```python
from build123d import *

# Parameters (mm, degrees)
BOSS_EXTRUDE1_DEPTH = 1
SKETCH2_W           = 2.9
SKETCH2_H           = 0.55
BOSS_EXTRUDE2_DEPTH = 10


with BuildPart() as part:
    # Sketch1 → Boss-Extrude1 (new, symmetric)
    with BuildSketch(Plane(origin=(0, 0, 0), x_dir=(1, 0, 0), z_dir=(0, 1, 0))):
        Polygon((40.414518843, 0), (20.207259422, 35), (-20.207259422, 35), (-40.414518843, 0), (-20.207259422, -35), (20.207259422, -35), align=None)
    extrude(amount=BOSS_EXTRUDE1_DEPTH, both=True)

    # Sketch2 → Boss-Extrude2 (add, symmetric)
    with BuildSketch(Plane(origin=(0, 0, 0), x_dir=(0, 0, -1), z_dir=(1, 0, 0))):
        Polygon((6.05, 5.45), (6.05, 4.05), (8.55, 1.55), (11.45, 1.55), (13.95, 4.05), (13.95, 5.45), align=None)
        Polygon((-6.05, 5.45), (-6.05, 4.05), (-8.55, 1.55), (-11.45, 1.55), (-13.95, 4.05), (-13.95, 5.45), align=None)
        with Locations((-10, 1.275)):
            Rectangle(SKETCH2_W, SKETCH2_H)
        with Locations((10, 1.275)):
            Rectangle(SKETCH2_W, SKETCH2_H)
    extrude(amount=BOSS_EXTRUDE2_DEPTH, both=True)


solid = part.part
```
Input: part model. Units: mm. Frame: model coordinates. A direction names the side the tool comes from. Round coordinates to 2 decimals unless told otherwise and drop trailing zeros. Loops run counter-clockwise (first coordinate to the right, second up) from the corner with the lowest first, then second, coordinate; pieces in that order, holes last. Notation, with made-up numbers: (31.5, 56) -> (57.5, 56) arc R22 cw to (57.5, 91) -> close; hole circle Ø5 at (89, 79). An arc over 180 degrees is marked (long way). Use one line per item in the form item = value. Start each with the question number.
Item 1: Contact query for flat-ended pins moving along their axis: pin 1 Ø1.3 at (y, z) = (3.5, 9) entering from +X; pin 2 Ø0.7 at (x, y) = (4, 4.5) entering from -Z; pin 3 Ø10 at (x, z) = (-10, 1) entering from +Y; pin 4 Ø3 at (x, y) = (13, 3.5) entering from +Z. Output: stop coordinate, or through.
Item 2: Mould query, pull axis Y, two halves, no side actions, for faces 1 (the face through (0, 0, -35)), 2 (the face through (-0.1, 2.8, -12.7)), 3 (the face through (0.1, 2.8, 12.7)), 4 (the face through (-1, -1, 0)). Classes: pulls with the +Y half, pulls with the -Y half, needs draft (parallel to the pull), parting line crosses it, or undercut.
Item 3: Section query C-C on z = -22. Return the cut outline in (x, y), then the cut area to 3 significant figures.
Item 4: Material intervals for L1, parallel to Z at x = 1, y = 4.25; L2, parallel to Z at x = -5, y = 1.5; L3, parallel to Y at x = -12, z = -9, sorted ascending. Write a range as from..to.
Item 5: Section query B-B on x = -12.5. Return the cut outline in (y, z), then the cut area to 3 significant figures.
Item 6: Set-up query: faces 5 (the face through (-30.45, 0.01, 17.26)), 6 (the face through (-10, 4, -10)), 7 (the face through (-0.1, 2.8, -7.3)), 8 (the face through (10, 4, 10)). Return all of +Z, -Z, +X, -X, +Y, -Y with unobstructed straight access to the full face (end or side cutting, diameter ignored); none if empty.
Item 7: Section query A-A on y = 0. Return the cut outline in (x, z), then the cut area to 3 significant figures.
Ans:
q1.pin_1 = 10
q1.pin_2 = -13.95
q1.pin_3 = 1
q1.pin_4 = through
q2.face_1 = needs draft
q2.face_2 = undercut
q2.face_3 = undercut
q2.face_4 = pulls with the -Y half
q3.outline = (-27.71, -1) -> (27.71, -1) -> (27.71, 1) -> (-27.71, 1) -> close
q3.area = 111 mm^2
q4.L1 = -13.95..-6.05, 6.05..13.95
q4.L2 = -11.45..-8.55, 8.55..11.45
q4.L3 = -1..1
q5.outline = (-1, -35) -> (1, -35) -> (1, 35) -> (-1, 35) -> close
q5.area = 140 mm^2
q6.face_5 = +Z, -X, +Y, -Y
q6.face_6 = +Z, -Z, -X, +Y
q6.face_7 = +X, -X
q6.face_8 = +Z, -Z, +X, +Y
q7.outline = (-40.41, 0) -> (-20.21, -35) -> (20.21, -35) -> (40.41, 0) -> (20.21, 35) -> (-20.21, 35) -> close
q7.area = 4,240 mm^2
